```python
from build123d import *

# Parameters (mm, degrees)
F1_DEPTH = 41
F3_DEPTH = 25


with BuildPart() as f1:
    # F0 (on Front) → F1 (new body)
    with BuildSketch(Plane.XZ):
        Polygon((15.397609, 0), (0, 0), (0, -5.324407), (5.036601, -5.324407), (5.036601, -25.664302), (55.889241, -25.664302), (55.889241, -5.324407), (60.976975, -5.324407), (60.976975, 0), (45.510266, 0), (45.510266, -5.324407), (50.597999, -5.324407), (50.597999, -21.187095), (10.17818, -21.187095), (10.17818, -5.324407), (15.397609, -5.324407), align=None)
    extrude(amount=F1_DEPTH)

    # F2 (on face) → F3 (cut)
    with BuildSketch(Plane.XY.offset(-21.187095)):
        with BuildLine():
            ThreePointArc((35.350505, -7.902889), (30.443043, -2.995427), (25.535582, -7.902889))
            Line((25.535582, -7.902889), (25.535582, -32.540347))
            ThreePointArc((25.535582, -32.540347), (30.443043, -37.447809), (35.350505, -32.540347))
            Line((35.350505, -32.540347), (35.350505, -7.902889))
        make_face()
    extrude(amount=-F3_DEPTH, mode=Mode.SUBTRACT)


solid = f1.part
```
The model under review builds one solid part; all positions refer to its coordinate system, in mm. A direction names the side the tool comes from. Round coordinates to 2 decimals unless told otherwise and drop trailing zeros. Write each loop counter-clockwise with the first axis right and the second up, starting at its lowest first coordinate (ties: lowest second). Pieces come first, ordered by that corner, then holes.
(1) We need section C-C on x = 13.5. Give the boundary of the cut face in (y, z), and give its area (3 significant figures).
(2) We need section A-A on y = -25. Give the boundary of the cut face in (x, z).
(3) We need section B-B on z = -3. Give the boundary of the cut face in (x, y).
(4) Mouldability with a two-part tool opening along Y and no side actions: class faces 1 (the flat face through (8, -20, 0)), 2 (the flat face through (30, -41, -22)), 3 (the cylindrical face through (30.551, -2.997, -23.394)), 4 (the cylindrical face through (30.335, -37.447, -23.394)) as +Y half, -Y half, draft (parallel to the pull), parting line (faces both ways), or undercut.
(5) Wall thickness on L1, parallel to X at y = -19, z = -13; L2, parallel to Z at x = 47, y = -32.5; L3, parallel to X at y = -13, z = -1.75: over which ranges is each line inside the solid? List them lowest first.
(6) We need section D-D on z = -23.25. Give the boundary of the cut face in (x, y), and give its area (3 significant figures).
(7) Insertion check: pin 1 (6 mm diameter, centred on x = 36.5, y = -17.5, fed in from +Z); pin 2 (4 mm diameter, centred on x = 1.5, y = -12.5, fed in from -Z); pin 3 (6 mm diameter, centred on y = -28.5, z = -18, fed in from +X); pin 4 (5.5 mm diameter, centred on x = 57.5, y = -26, fed in from -Z). Each pin has a flat end and moves straight along its axis. Give the tip position at first contact, or say it passes through.
(8) Machinability: for faces 5 (the flat face through (5.037, -20, -15)), 6 (the flat face through (10.178, -20, -13)), 7 (the flat face through (15.398, -20, -3)), which of the approach directions +Z, -Z, +X, -X, +Y, -Y give a long, thin tool a straight path to every point of the face, cutting with its end or side? Answer none if there is none.
Findings below:
1. outline: (-41, -25.66) - (0, -25.66) - (0, -21.19) - (-41, -21.19) - close; (-41, -5.32) - (0, -5.32) - (0, 0) - (-41, 0) - close
1. area: 402 mm2
2. outline: (0, -5.32) - (5.04, -5.32) - (5.04, -25.66) - (25.54, -25.66) - (25.54, -21.19) - (10.18, -21.19) - (10.18, -5.32) - (15.4, -5.32) - (15.4, 0) - (0, 0) - close; (35.35, -25.66) - (55.89, -25.66) - (55.89, -5.32) - (60.98, -5.32) - (60.98, 0) - (45.51, 0) - (45.51, -5.32) - (50.6, -5.32) - (50.6, -21.19) - (35.35, -21.19) - close
3. outline: (0, -41) - (15.4, -41) - (15.4, 0) - (0, 0) - close; (45.51, -41) - (60.98, -41) - (60.98, 0) - (45.51, 0) - close
4. face 1: draft
4. face 2: -Y half
4. face 3: undercut
4. face 4: undercut
5. L1: x = 5.04 to 10.18, 50.6 to 55.89
5. L2: z = -25.66 to -21.19, -5.32 to 0
5. L3: x = 0 to 15.4, 45.51 to 60.98
6. outline: (5.04, -41) - (55.89, -41) - (55.89, 0) - (5.04, 0) - close; hole (25.54, -32.54) arc R4.91 ccw to (35.35, -32.54) - (35.35, -7.9) arc R4.91 ccw to (25.54, -7.9) - close
6. area: 1,770 mm2
7. pin 1: stops at z = -21.19
7. pin 2: stops at z = -5.32
7. pin 3: stops at x = 55.89
7. pin 4: stops at z = -25.66
8. face 5: -Z, -X, +Y, -Y
8. face 6: +Y, -Y
8. face 7: +Z, +Y, -Y
